from build123d import *

# Parameters (mm, degrees)
CROQUIS1_R              = 9
SALIENTE_EXTRUIR1_DEPTH = 3
CROQUIS2_R              = 7
SALIENTE_EXTRUIR2_DEPTH = 27
CROQUIS4_R              = 3.75
SALIENTE_EXTRUIR3_DEPTH = 4
CROQUIS5_R              = 7
SALIENTE_EXTRUIR4_DEPTH = 9
CROQUIS7_R              = 7
SALIENTE_EXTRUIR5_DEPTH = 5
CHAFL_N1_SIZE           = 1.5


with BuildPart() as part:
    # Croquis1 → Saliente-Extruir1 (new body)
    with BuildSketch(Plane(origin=(0, 0, 0), x_dir=(1, 0, 0), z_dir=(0, 1, 0))):
        Circle(CROQUIS1_R)
    extrude(amount=SALIENTE_EXTRUIR1_DEPTH)

    # Croquis2 → Saliente-Extruir2 (add)
    with BuildSketch(Plane(origin=(0, 0, 0), x_dir=(1, 0, 0), z_dir=(0, 1, 0))):
        Circle(CROQUIS2_R)
    extrude(amount=SALIENTE_EXTRUIR2_DEPTH)

    # Croquis4 → Saliente-Extruir3 (add)
    with BuildSketch(Plane(origin=(0, 27, 0), x_dir=(1, 0, 0), z_dir=(0, 1, 0))):
        Circle(CROQUIS4_R)
    extrude(amount=SALIENTE_EXTRUIR3_DEPTH)

    # Croquis5 → Saliente-Extruir4 (add)
    with BuildSketch(Plane(origin=(0, 31, 0), x_dir=(1, 0, 0), z_dir=(0, 1, 0))):
        Circle(CROQUIS5_R)
    extrude(amount=SALIENTE_EXTRUIR4_DEPTH)

    # Croquis7 → Saliente-Extruir5 (add)
    with BuildSketch(Plane.XZ):
        Circle(CROQUIS7_R)
    extrude(amount=SALIENTE_EXTRUIR5_DEPTH)

    # Chaflán1
    chafl_n1_edges = [part.edges().sort_by_distance(p)[0] for p in [
        (-7, 40, 0),
    ]]
    chamfer(chafl_n1_edges, length=CHAFL_N1_SIZE)


solid = part.part
Work out the finished part from the listing and answer in its coordinate system (mm). A direction names the side the tool comes from. Give positions to 0.01 mm unless a question says otherwise; leave off trailing zeros. Order: outer loops, then holes, each group sorted by start corner. A loop starts at its lowest first (then second) coordinate and runs counter-clockwise, first axis right, second up. Notation, with made-up numbers: M 44,77.5 L 54,77.5 A31 ccw 54,111.5 Z; hole C 52,-33 d3. An arc over 180 degrees is marked long. Return JSON: item names as keys, results as strings.
Q1. The mould has two halves that part along Y. Classify faces 5 (the face through (0, -5, 0)), 6 (the face through (6.466, -2.465, -2.681)), 7 (the face through (-3.746, 28.972, -0.165)): pulls with the +Y half, pulls with the -Y half, needs draft (parallel to the pull), parting line crosses it, or undercut.
Answer below:
{"face 5": "pulls with the -Y half", "face 6": "needs draft", "face 7": "undercut"}
Q2. Each of these flat-tipped pins is pushed along its axis until it touches: pin 1 (5 mm diameter, centred on y = 30, z = -2.5, fed in from -X); pin 2 (10 mm diameter, centred on x = -7, y = 27, fed in from -Z); pin 3 (4 mm diameter, centred on y = 8, z = 6, fed in from -X). Where does it stop, or does it pass through?
Answer below:
{"pin 1": "stops at x = -7", "pin 2": "stops at z = -6.71", "pin 3": "stops at x = -5.74"}
Q3. Find section B-B, the plane x = 0. Write down the section's boundary in (y, z), and give its area (3 significant figures).
Answer below:
{"outline": "M -5,-7 L 0,-7 L 0,-9 L 3,-9 L 3,-7 L 27,-7 L 27,-3.75 L 31,-3.75 L 31,-7 L 38.5,-7 L 40,-5.5 L 40,5.5 L 38.5,7 L 31,7 L 31,3.75 L 27,3.75 L 27,7 L 3,7 L 3,9 L 0,9 L 0,7 L -5,7 Z", "area": "614 mm^2"}
Q4. Find section A-A, the plane z = 0. Write down the section's boundary in (x, y), and give its area (3 significant figures).
Answer below:
{"outline": "M -9,0 L -7,0 L -7,-5 L 7,-5 L 7,0 L 9,0 L 9,3 L 7,3 L 7,27 L 3.75,27 L 3.75,31 L 7,31 L 7,38.5 L 5.5,40 L -5.5,40 L -7,38.5 L -7,31 L -3.75,31 L -3.75,27 L -7,27 L -7,3 L -9,3 Z", "area": "614 mm^2"}
Q5. Find the intervals of material crossed by line 1 along Y through (x, z) = (3.5, 6.5); line 2 along X through (y, z) = (14.5, -5); line 3 along Z through (x, y) = (-4.5, 33), in increasing order. Write a range as [from, to].
Answer below:
{"line 1": "y = [0, 3]", "line 2": "x = [-4.9, 4.9]", "line 3": "z = [-5.36, 5.36]"}
Q6. Find section C-C, the plane y = 5.5. Write down the section's boundary in (x, z), and give its area (3 significant figures).
Answer below:
{"outline": "C 0,0 d14", "area": "154 mm^2"}
Q7. Which of the six approach directions +Z, -Z, +X, -X, +Y, -Y give full straight-line access (tool end or side, diameter ignored) to faces 1 (the face through (6.466, 14.832, 2.681)), 2 (the face through (0, 0, 7.3)), 3 (the face through (0, 40, 0)), 4 (the face through (3, 27, 3))?
Answer below:
{"face 1": "+Y", "face 2": "-Y", "face 3": "+Z, -Z, +X, -X, +Y", "face 4": "none"}
